Geometry: see drawing. Coordinates: mm, zero at the bounding-box minimum. Give positions to 0.01 mm unless a question says otherwise; leave off trailing zeros. Loops run counter-clockwise (first coordinate to the right, second up) from the corner with the lowest first, then second, coordinate; pieces in that order, holes last. Notation, with made-up numbers: M 64,62 L 101,62 A9 ccw 101,75 Z; hole C -32.75,89.5 d9. An arc over 180 degrees is marked long. Answer in a Markdown table with one row per item.
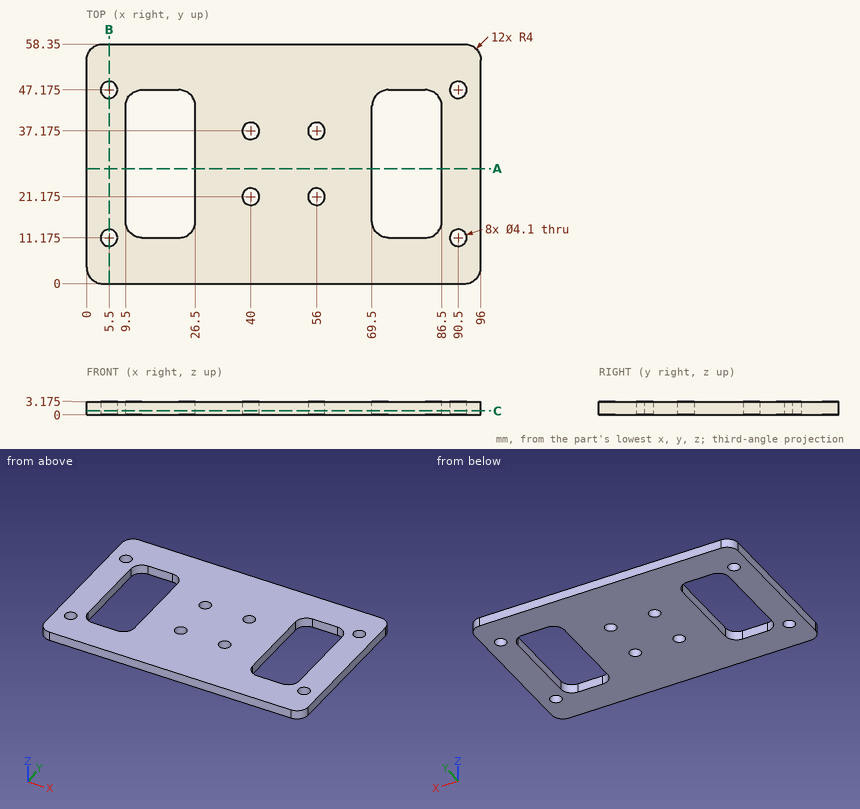
1) Pin query (flat end, axial travel): pin 1 Ø3.5 at (x, y) = (90.5, 11.175) entering from -Z; pin 2 Ø4.5 at (x, y) = (5.5, 47.175) entering from -Z. Return the tip coordinate at first contact, or that it passes through.
Reply:
| item | result |
|---|---|
| pin 1 | passes through |
| pin 2 | stops at z = 0 |
2) Section A-A, the plane y = 28. Return loops of the section in (x, z) (3 decimals), then the cut area to 3 significant figures.
Reply:
| item | result |
|---|---|
| outline | M 0,0 L 9.5,0 L 9.5,3.175 L 0,3.175 Z; M 26.5,0 L 69.5,0 L 69.5,3.175 L 26.5,3.175 Z; M 86.5,0 L 96,0 L 96,3.175 L 86.5,3.175 Z |
| area | 197 mm² |
3) Section B-B, the plane x = 5.5. Return loops of the section in (y, z) (3 decimals), then the cut area to 3 significant figures.
Reply:
| item | result |
|---|---|
| outline | M 0,0 L 9.125,0 L 9.125,3.175 L 0,3.175 Z; M 13.225,0 L 45.125,0 L 45.125,3.175 L 13.225,3.175 Z; M 49.225,0 L 58.35,0 L 58.35,3.175 L 49.225,3.175 Z |
| area | 159 mm² |
4) Material intervals for L1, parallel to Y at x = 40, z = 2.4 (3 decimals); L2, parallel to X at y = 25.5, z = 0.6; L3, parallel to Y at x = 90.5, z = 1.75 (3 decimals), sorted ascending.
Reply:
| item | result |
|---|---|
| L1 | y = 0 to 19.125, 23.225 to 35.125, 39.225 to 58.35 |
| L2 | x = 0 to 9.5, 26.5 to 69.5, 86.5 to 96 |
| L3 | y = 0 to 9.125, 13.225 to 45.125, 49.225 to 58.35 |
5) Section C-C, the plane z = 0.95. Count the separate pieces of the cut face and the enclosed holes in it, then the cut area to 3 significant figures.
Reply:
| item | result |
|---|---|
| separate pieces | 1 |
| enclosed holes | 10 |
| area | 4,290 mm² |
